Autodesk Inventor part; units mm, degrees
ref_plane "YZ Plane" through (0, 0, 0) normal (1, 0, 0) x (0, 1, 0)
ref_plane "XZ Plane" through (0, 0, 0) normal (0, 1, 0) x (-1, 0, 0)
ref_plane "XY Plane" through (0, 0, 0) normal (0, 0, 1) x (1, 0, 0)
sketch "Sketch1" plane through (0, 0, 0) normal (0, 1, 0) x (-1, 0, 0)
  line L0 (332.74, 139.7) -> (-332.74, 139.7)
  line L1 (-332.74, 139.7) -> (-332.74, -139.7)
  line L2 (-332.74, -139.7) -> (332.74, -139.7)
  line L3 (332.74, -139.7) -> (332.74, 139.7)
  line L4 (332.74, 139.7) -> (-332.74, -139.7) construction
  line L5 (-332.74, 139.7) -> (332.74, -139.7) construction
  point P0 (0, 0)
  dimension "d0" = 665.48
  dimension "d1" = 279.4
extrude "Extrusion1" add sketch "Sketch1" along normal blind 19.05
sketch "Sketch2" plane through (0, 19.05, 0) normal (0, 1, 0) x (1, 0, 0)
  circle A0 centre (73.2058, 76.2) radius 50.8
  circle A1 centre (-104.14, -139.7) radius 38.1
  line L0 (-332.74, -139.7) -> (332.74, -139.7)
  line L1 (332.74, -139.7) -> (332.74, 139.7)
  line L2 (332.74, 139.7) -> (-332.74, 139.7)
  line L3 (-332.74, 139.7) -> (-332.74, -139.7)
  circle A2 centre (-104.14, -139.7) radius 12.7
  circle A3 centre (73.2058, 76.2) radius 14.859
  point P0 (0, 0)
  dimension "d12" = 101.6
  dimension "d13" = 76.2
  dimension "d27" = 25.4
  dimension "d28" = 29.718
sketch "Sketch4" plane through (-332.74, 0, 139.7) normal (0, 0, 1) x (1, 0, 0)
  line L0 (0, 0) -> (665.48, 0)
  line L1 (665.48, 0) -> (665.48, 19.05)
  line L2 (0, 19.05) -> (665.48, 19.05)
  line L3 (0, 0) -> (0, 19.05)
  point P0 (332.74, 0)
extrude "Extrusion3" add sketch "Sketch4" along normal blind 38.1
sketch "Sketch5" plane through (0, 19.05, 0) normal (0, 1, 0) x (1, 0, 0)
  line L0 (-332.74, -177.8) -> (-161.29, -177.8)
  line L1 (-161.29, -177.8) -> (-161.29, -127)
  line L2 (-161.29, -127) -> (-332.74, -127)
  line L3 (-332.74, -127) -> (-332.74, -177.8)
  line L4 (332.74, -177.8) -> (-48.2601, -177.8)
  line L5 (-48.2601, -177.8) -> (-48.2601, -127)
  line L6 (-48.2601, -127) -> (332.74, -127)
  line L7 (332.74, -127) -> (332.74, -177.8)
  line L8 (332.74, -177.8) -> (-48.2601, -177.8)
  line L9 (-48.2601, -177.8) -> (-48.2601, -127)
  line L10 (-48.2601, -127) -> (332.74, -127)
  line L11 (332.74, -127) -> (332.74, -177.8)
  point P0 (0, 0)
  dimension "d18" = 171.45
  dimension "d19" = 50.8
extrude "Extrusion5" cut sketch "Sketch5" against normal blind 50.8
sketch "Sketch6" plane through (-332.74, 0, -139.7) normal (-1, 0, 0) x (0, 0, 1)
  line L0 (266.7, 0) -> (266.7, 19.05)
  line L1 (0, 19.05) -> (266.7, 19.05)
  line L2 (0, 0) -> (0, 19.05)
  line L3 (0, 0) -> (266.7, 0)
  point P0 (139.7, 0)
extrude "Extrusion6" add sketch "Sketch6" along normal blind 53.975
sketch "Sketch7" plane through (-386.715, 0, -139.7) normal (-1, 0, 0) x (0, 0, 1)
  line L0 (266.7, 19.05) -> (0, 19.05)
  line L1 (266.7, 19.05) -> (147.066, 19.05)
  line L2 (0, 0) -> (147.066, 0)
  line L3 (147.066, 0) -> (147.066, 19.05)
  line L4 (147.066, 19.05) -> (0, 19.05)
  line L5 (0, 19.05) -> (0, 0)
  point P0 (139.7, 0)
  dimension "d24" = 119.634
extrude "Extrusion7" add sketch "Sketch7" along normal blind 19.05
properties part number "Robot Shooter Support Wall" material "Wood (Birch)"
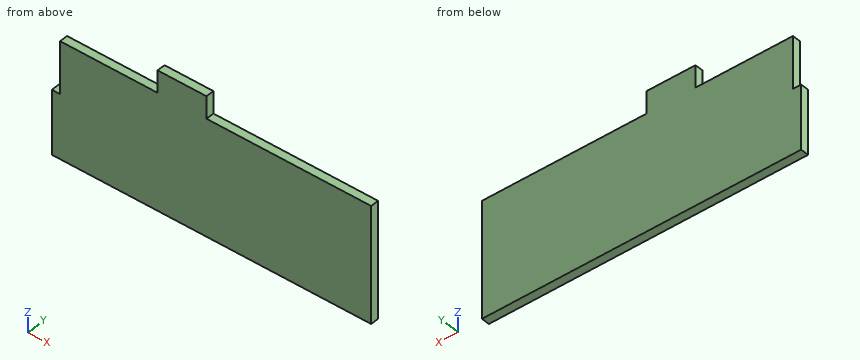
Input: part model. Units: mm. Frame: model coordinates. Coordinates: 2 decimals unless noted, no trailing zeros. Loops run counter-clockwise (first coordinate to the right, second up) from the corner with the lowest first, then second, coordinate; pieces in that order, holes last.
(1) Section A-A on y = 9.5. Return the cut outline in (x, z) (3 decimals), then the cut area to 3 significant figures.
(2) Section C-C on x = 213. Return the cut outline in (y, z), then the cut area to 3 significant figures.
(3) First-contact query: pin 1 Ø1 at (x, y) = (68, 16) entering from +Z; pin 2 Ø5.5 at (y, z) = (11.5, 66) entering from -X (3 decimals). Flat tips, straight axial feed; report the tip coordinate or a pass-through.
(4) Section B-B on z = 29. Return the cut outline in (x, y) (3 decimals).
(5) Material intervals for probe 1 along Z at (x, y) = (-36, 8); probe 2 along X at (y, z) = (17.25, 26) (3 decimals); probe 3 along X at (y, z) = (14, 151.5), sorted ascending.
Data:
1. outline: (-405.765, -139.7) - (332.74, -139.7) - (332.74, 127) - (-48.26, 127) - (-48.26, 177.8) - (-161.29, 177.8) - (-161.29, 127) - (-386.715, 127) - (-386.715, 7.366) - (-405.765, 7.366) - close
1. area: 200,000 mm2
2. outline: (0, -139.7) - (19.05, -139.7) - (19.05, 127) - (0, 127) - close
2. area: 5,080 mm2
3. pin 1: stops at z = 127
3. pin 2: stops at x = -386.715
4. outline: (-386.715, 0) - (332.74, 0) - (332.74, 19.05) - (-386.715, 19.05) - close
5. probe 1: z = -139.7 to 127
5. probe 2: x = -386.715 to 332.74
5. probe 3: x = -161.29 to -48.26
